Work out the finished part from the listing and answer in its coordinate system (mm). A direction names the side the tool comes from. Round coordinates to 2 decimals unless told otherwise and drop trailing zeros. Write each loop counter-clockwise with the first axis right and the second up, starting at its lowest first coordinate (ties: lowest second). Pieces come first, ordered by that corner, then holes.
from build123d import *

# Parameters (mm, degrees)
SKETCH_1_W             = 110
SKETCH_1_H             = 50
EXTRUDE_1_DEPTH        = 5
SKETCH_2_R             = 3
EXTRUDE_2_DEPTH        = 7.5
HOLE_WIZARD_M4_1_D     = 3.3
HOLE_WIZARD_M4_1_DEPTH = 5
HOLE_WIZARD_M4_1_TIP   = 0.991420021
SKETCH_6_W             = 110
SKETCH_6_H             = 25
EXTRUDE_3_DEPTH        = 6.5
FILLET_1_R             = 10
CHAMFER_1_SIZE         = 5
FILLET_2_R             = 10


with BuildPart() as part:
    # 草图1 → 凸台-拉伸1 (new body)
    with BuildSketch(Plane.XY):
        Rectangle(SKETCH_1_W, SKETCH_1_H)
    extrude(amount=EXTRUDE_1_DEPTH)

    # 草图2 → 凸台-拉伸2 (add)
    with BuildSketch(Plane.XY.offset(5)):
        with Locations((-48, 0)):
            Circle(SKETCH_2_R)
        with Locations((48, 0)):
            Circle(SKETCH_2_R)
        with BuildLine():
            Line((-38, 16.5), (38, 16.5))
            ThreePointArc((38, 16.5), (41.535533906, 15.035533906), (43, 11.5))
            Line((43, 11.5), (43, -11.5))
            ThreePointArc((43, -11.5), (41.535533906, -15.035533906), (38, -16.5))
            Line((38, -16.5), (-38, -16.5))
            ThreePointArc((-38, -16.5), (-41.535533906, -15.035533906), (-43, -11.5))
            Line((-43, -11.5), (-43, 11.5))
            ThreePointArc((-43, 11.5), (-41.535533906, 15.035533906), (-38, 16.5))
        make_face()
    extrude(amount=EXTRUDE_2_DEPTH)

    # M4 螺纹孔1
    with Locations(Plane.XY.offset(12.5)):
        with Locations((48, 0), (-48, 0)):
            Hole(HOLE_WIZARD_M4_1_D / 2, depth=HOLE_WIZARD_M4_1_DEPTH)
            with Locations((0, 0, -(HOLE_WIZARD_M4_1_DEPTH + HOLE_WIZARD_M4_1_TIP / 2))):  # 118° drill point
                Cone(0, HOLE_WIZARD_M4_1_D / 2, HOLE_WIZARD_M4_1_TIP, mode=Mode.SUBTRACT)

    # 草图6 → 凸台-拉伸3 (add)
    with BuildSketch(Plane(origin=(0, 0, 0), x_dir=(-1, 0, 0), z_dir=(0, 0, -1))):
        with Locations((0, 12.5)):
            Rectangle(SKETCH_6_W, SKETCH_6_H)
    extrude(amount=EXTRUDE_3_DEPTH)

    # 圆角1
    fillet_1_edges = [part.edges().sort_by_distance(p)[0] for p in [
        (55, -25, 2.5),
        (-55, -25, 2.5),
        (-55, 25, -0.75),
        (55, 25, -0.75),
    ]]
    fillet(fillet_1_edges, radius=FILLET_1_R)

    # 倒角1
    chamfer_1_edges = [part.edges().sort_by_distance(p)[0] for p in [
        (-55, 7.5, -6.5),
        (0, 25, -6.5),
        (55, 7.5, -6.5),
        (-52.071067812, 22.071067812, -6.5),
        (52.071067812, 22.071067812, -6.5),
    ]]
    chamfer(chamfer_1_edges, length=CHAMFER_1_SIZE)

    # 圆角2
    # the kernel refuses this fillet: 10 mm, written as the material it adds along each edge
    with BuildSketch(Plane(origin=(55, 0, 0), x_dir=(0, 0, -1), z_dir=(-1, 0, 0))) as fillet_2_piece_1_section:
        with BuildLine():
            CenterArc((10, 9.367496998), FILLET_2_R, 180, 69.512684885)
            Line((0, 9.367496998), (-0.2, 9.367496998))
            Line((-0.2, 9.367496998), (-0.2, 0))
            Line((-0.2, 0), (0, -0.2))
            ThreePointArc((0, -0.2), (3.25, -0.2), (6.43, -0.18734994))
            Line((6.43, -0.18734994), (6.5, 0))
        make_face()
    fillet_2_piece_1 = extrude(amount=110, mode=Mode.PRIVATE)
    fillet_2_piece_1 = split(fillet_2_piece_1, bisect_by=Plane(origin=(-27.428646518, -2.275588703, -29.071353482), z_dir=(0.7071067811865476, 0, 0.7071067811865476)), keep=Keep.TOP, mode=Mode.PRIVATE)
    fillet_2_piece_1 = split(fillet_2_piece_1, bisect_by=Plane(origin=(27.428646518, -2.275588703, -29.071353482), z_dir=(-0.7071067811865476, 0, 0.7071067811865476)), keep=Keep.TOP, mode=Mode.PRIVATE)
    add(fillet_2_piece_1)


solid = part.part
Q1. Given pin 1 (4 mm diameter, centred on x = 17, z = 10.5, fed in from +Y); pin 2 (2 mm diameter, centred on x = -16, z = 10, fed in from -Y); pin 3 (3 mm diameter, centred on x = 48, y = 0, fed in from +Z), each flat-ended and moving along its own axis, determine where each tip first touches the part or whether it passes through.
Q2. Find section B-B (x = -21.5). Determine the outline of the cut face in (y, z), plus the area to 3 significant figures.
Q3. A tool of negligible diameter and unlimited length cuts with its end or side. For faces 1 (the face through (-1, 16.5, 9)), 2 (the face through (-1, 17, 5)), 3 (the face through (-1, -17, 0)), 4 (the face through (-46.7, -1.3, 12.5)), 5 (the face through (1, -16.5, 9)), from which of +Z, -Z, +X, -X, +Y, -Y can it reach the whole face along a straight path? Write none if from no direction.
Q4. Find section C-C (z = 4). Determine the outline of the cut face in (x, y), plus the area to 3 significant figures.
Q5. Find section D-D (x = -44). Determine the outline of the cut face in (y, z).
Q6. Find the intervals of material crossed by L1, parallel to Y at x = -48, z = 9.5; L2, parallel to Y at x = -37, z = 8.25; L3, parallel to Z at x = 18, y = -20, in increasing order.
Q7. Find section A-A (z = 9.25). Determine the outline of the cut face in (x, y).
Report:
1. pin 1: stops at y = 16.5
1. pin 2: stops at y = -16.5
1. pin 3: stops at z = 7.41
2. outline: (-25, 0) - (-9.37, 0) arc R10 cw to (0, -6.5) - (20, -6.5) - (25, -1.5) - (25, 5) - (16.5, 5) - (16.5, 12.5) - (-16.5, 12.5) - (-16.5, 5) - (-25, 5) - close
2. area: 664 mm2
3. face 1: +Z, +X, -X, +Y
3. face 2: +Z
3. face 3: -Z, +X, -X, -Y
3. face 4: +Z, +X, -X, +Y, -Y
3. face 5: +Z, +X, -X, -Y
4. outline: (-55, -15) arc R10 ccw to (-45, -25) - (45, -25) arc R10 ccw to (55, -15) - (55, 15) arc R10 ccw to (45, 25) - (-45, 25) arc R10 ccw to (-55, 15) - close
4. area: 5,410 mm2
5. outline: (-25, 0) - (-9.37, 0) arc R10 cw to (0, -6.5) - (20, -6.5) - (25, -1.5) - (25, 5) - (-25, 5) - close
6. L1: y = -3 to -1.65, 1.65 to 3
6. L2: y = -16.5 to 16.5
6. L3: z = 0 to 5
7. outline: circle Ø6 at (-48, 0); (-43, -11.5) arc R5 ccw to (-38, -16.5) - (38, -16.5) arc R5 ccw to (43, -11.5) - (43, 11.5) arc R5 ccw to (38, 16.5) - (-38, 16.5) arc R5 ccw to (-43, 11.5) - close; circle Ø6 at (48, 0); hole circle Ø3.3 at (-48, 0); hole circle Ø3.3 at (48, 0)
